Verification items for the finished model (mm, model axes). A direction names the side the tool comes from. Round coordinates to 2 decimals unless told otherwise and drop trailing zeros. Write each loop counter-clockwise with the first axis right and the second up, starting at its lowest first coordinate (ties: lowest second). Pieces come first, ordered by that corner, then holes. Notation, with made-up numbers: M 88,-29 L 97,-29 A28 ccw 97,-1 Z; hole C -6.75,-9 d9. An arc over 180 degrees is marked long. One line per question, with ' | ' between items.
Autodesk Inventor part; units mm, degrees
ref_plane "Work Plane1" through (10.95, 0, 0) normal (0, 0, -1) x (1, 0, 0)
ref_plane "YZ Plane" through (0, 0, 0) normal (1, 0, 0) x (0, 1, 0)
ref_plane "XZ Plane" through (0, 0, 0) normal (0, 1, 0) x (-1, 0, 0)
sketch "Sketch1" plane through (0, 0, 0) normal (0, 0, 1) x (1, 0, 0)
  line L0 (-3.2004, 0) -> (-3.2004, 3.8156)
  line L1 (0, 6.096) -> (0, 3.175)
  line L2 (4.1148, 3.175) -> (19.05, 3.175)
  line L3 (19.05, 3.175) -> (19.05, 0)
  line L4 (19.05, 0) -> (-3.2004, 0)
  arc A0 (0, 6.096) -> (-1.9368, 6.5254) centre (-1.016, 6.096) ccw
  line L5 (0, -1.4605) -> (0, 8.7631)
  line L6 (-7.6505, 0) -> (23.5001, 0)
  line L7 (0, 3.175) -> (0.0001, 3.175)
  line L8 (0.0001, 3.175) -> (0.0001, 3.175)
  line L9 (0.0001, 3.175) -> (2.2098, 3.175)
  line L10 (2.2098, 3.175) -> (4.1148, 3.175)
  line L11 (-3.2004, 3.8156) -> (-1.9368, 6.5254)
  line L12 (0.0001, 3.175) -> (4.1148, 3.175) construction
  line L13 (4.1148, 3.175) -> (4.1148, 0) construction
  dimension "d0" = 1.016
  dimension "d1" = 19.05
  dimension "d2" = 14.9352
  dimension "d3" = 14.224
  dimension "d4" = 6.35
  dimension "d5" = 3.2004
  dimension "d15" = 6.35
  dimension "d16" = 6.35
  dimension "d17" = 0.0001
  dimension "d18" = 1.905
  dimension "d19" = 25
revolve "Body" add sketch "Sketch1" angle 360 about axis through (19.05, 0, 0) along (-1, 0, 0)
sketch "Sketch2" plane through (0, 0, 0) normal (1, 0, 0) x (0, 0, -1)
  line L0 (4.7625, 2.7496) -> (4.7625, -2.7496)
  line L1 (4.7625, -2.7496) -> (0, -5.4993)
  line L2 (0, -5.4993) -> (-4.7625, -2.7496)
  line L3 (-4.7625, -2.7496) -> (-4.7625, 2.7496)
  line L4 (-4.7625, 2.7496) -> (0, 5.4993)
  line L5 (0, 5.4993) -> (4.7625, 2.7496)
  point P0 (0, 0)
  point P1 (0, 0)
  dimension "d23" = 9.525
extrude "Head" add sketch "Sketch2" against normal blind 7.112
sketch "Sketch3" plane through (0, 0, 0) normal (0, 0, 1) x (1, 0, 0)
  line L0 (-7.112, 4.7625) -> (-7.112, 5.4993)
  line L1 (-7.112, 5.4993) -> (-6.6866, 5.4993)
  line L2 (-6.6866, 5.4993) -> (-7.112, 4.7625)
  line L3 (-8.0513, 0) -> (-1.476, 0)
  line L4 (-7.112, 5.4993) -> (-7.112, 2.7496)
  line L5 (-2.4153, 5.4993) -> (-7.112, 5.4993)
  point P0 (-7.112, 2.7496)
  dimension "d8" = 30
  dimension "d22" = 9.525
revolve "Chamfer1" cut sketch "Sketch3" angle 360 about axis through (-10, 0, 0) along (1, 0, 0)
thread "Thread"
chamfer "Chamfer2" distance 0.7791 distance2 0.7791 1 edges at (19.05, -3.175, 0) measured on face at (19.05, -0.6414, -1.6914)
ref_plane "Work Plane1" through (10.95, 0, 0) normal (0, 0, -1) x (1, 0, 0)
equation "\"d0\" = PHH"
equation "\"d1\" = NLG"
equation "\"d2\" = GEL"
equation "\"d3\" = LADI"
equation "\"d4\" = GD"
equation "\"d5\" = 0.45 * KOH"
equation "\"d15\" = SD2"
equation "\"d16\" = BDM"
equation "\"d18\" = GAL"
equation "\"d19\" = KEWI"
equation "\"d23\" = SW"
equation "\"d6\" = KOH"
equation "\"d8\" = ANG1"
equation "\"d22\" = SW0"
equation "\"d10\" = GEL"
equation "\"d13\" = -0.5 * SPD + 0.5 * GD"
equation "\"d14\" = GUL"
equation "\"NLG\" = 19.05"
equation "\"GD\" = NND"
equation "\"BDM\" = NND"
equation "\"KOH\" = 7.112"
equation "\"GEL\" = 14.9352"
equation "\"LADI\" = 14.224"
equation "\"SW\" = 9.525"
equation "\"PHH\" = 1.016"
equation "\"SW0\" = SW"
equation "\"SPD\" = 4.79184"
equation "\"SD2\" = NND"
equation "\"SD\" = 0"
equation "\"ANG1\" = 30deg"
equation "\"KEWI\" = 25deg"
equation "\"GAL\" = 1.905"
equation "\"GUL\" = 0.77908"
equation "\"THREADDIA\" = 6.35"
equation "\"SDH\" = SW"
equation "\"TOA\" = 30deg"
equation "\"NND\" = 6.35"
equation "\"E0\" = 1.155 * SW"
equation "\"GD1\" = 4.79184"
properties part number "am-1271" material "Steel, Mild"
1. Go/stop test with flat-tipped pins: P1, Ø2, axis at x = 7.5, z = -2, coming from the +Y side; P2, Ø4, axis at x = 7.5, z = -4, coming from the +Y side; P3, Ø1, axis at x = -3, y = -5.5, coming from the +Z side. Record where each tip stops, or that it passes through.
Results:
P1: stops at y = 3.01 | P2: stops at y = 2.47 | P3: stops at z = 0.86
2. Thickness scan on line 1 (X direction, y = 3.5, z = -2); line 2 (X direction, y = -1.5, z = 5.25); line 3 (Y direction, x = -2.5, z = 2.5). Record the ranges inside material, lowest first.
Results:
line 1: x = -7.11 to 0 | line 2: x = -2.43 to 0 | line 3: y = -4.69 to 4.69
3. Section check A-A, the plane x = 4.5. Record the cut outline in (y, z) (3 decimals), then the cut area to 3 significant figures.
Results:
outline: C 0,0 d6.35 | area: 31.7 mm2
4. Tool access check on faces 1 (the face through (0, 3, 3)), 2 (the face through (-4.731, -4.144, 2.348)), 3 (the face through (-4.73, 4.11, 2.41)), 4 (the face through (-4.731, 4.144, -2.348)). Record the directions out of +Z, -Z, +X, -X, +Y, -Y that give a thin tool (end or side, any length) a straight path to the whole face; none if there is none.
Results:
face 1: +X | face 2: +Z, -X, -Y | face 3: +Z, -X, +Y | face 4: -Z, -X, +Y
5. Section check B-B, the plane x = -1.25. Record the cut outline in (y, z).
Results:
outline: C 0,0 d14.17
